Can you work these out from the model? Positions are in its coordinate system, mm. A direction names the side the tool comes from. Give positions to 0.01 mm unless a question says otherwise; leave off trailing zeros. Loops run counter-clockwise (first coordinate to the right, second up) from the corner with the lowest first, then second, coordinate; pieces in that order, holes last. Notation, with made-up numbers: (-22, 1.5) -> (-10, 1.5) arc R20 cw to (-10, 7.5) -> close; hole circle Ø10 at (45.5, 72.5). An arc over 180 degrees is marked (long way). Use CSV: the item, a comma, the result in double quotes.
from build123d import *

# Parameters (mm, degrees)
F3_DEPTH  = 6.501
F5_DEPTH  = 50
F8_W      = 9.4140861183
F8_H      = 9.8263791297
F9_DEPTH  = 25
F12_W     = 14.8912463337
F12_H     = 11.3480030559
F13_DEPTH = 25


with BuildPart() as f1:
    # F0 (on Front) → F1 (revolve)
    with BuildSketch(Plane.XZ):
        Polygon((-12, 5), (-22.5, 5), (-22.5, 5.6), (-23, 5.6), (-24.5, 5), (-24.5, 2.5), (-10, 2.5), (-8, 4.5), (-1, 4.5), (0, 5.5), (0, 6.5), (-10.5, 6.5), align=None)
    revolve(axis=Axis((-0.2357512317, 0, 0), (1, 0, 0)))

    # F2 (on Front) → F3 (cut, through all)
    with BuildSketch(Plane.XZ):
        with BuildLine():
            Line((0, 2.4), (-3.6575932294, 1.75))
            ThreePointArc((-3.6575932294, 1.75), (-7.7, 0), (-3.6575932294, -1.75))
            Line((-3.6575932294, -1.75), (0, -2.4))
            Line((0, -2.4), (0, 2.4))
        make_face()
    extrude(amount=-F3_DEPTH, mode=Mode.SUBTRACT)

    # F4 (on Top) → F5 (cut, symmetric)
    with BuildSketch(Plane.XY):
        with BuildLine():
            Line((-15.5885848908, 1.2395342523), (-24.5, 2.4))
            Line((-24.5, 2.4), (-24.5, -2.4))
            Line((-24.5, -2.4), (-15.5885848908, -1.2395342523))
            ThreePointArc((-15.5885848908, -1.2395342523), (-14.5, 0), (-15.5885848908, 1.2395342523))
        make_face()
    extrude(amount=F5_DEPTH, both=True, mode=Mode.SUBTRACT)

    # F8 (on 3pt) → F9 (cut)
    with BuildSketch(Plane(origin=(-0.2560212454, -0.0401067578, -5.558750384), x_dir=(0.9989411003, -0.0003319376, -0.046006173), z_dir=(0.0460073704, 0.0072072396, 0.9989151003))):
        with Locations((-24.0980023518, 1.025695703)):
            Rectangle(F8_W, F8_H)
    extrude(amount=-F9_DEPTH, mode=Mode.SUBTRACT)

    # F12 (on 3pt) → F13 (cut)
    with BuildSketch(Plane(origin=(-0.2560212454, -0.0401067578, 5.558750384), x_dir=(0.9989411003, -0.0003319376, 0.046006173), z_dir=(0.0460073704, 0.0072072396, -0.9989151003))):
        with Locations((-25.9663937613, -0.8096385282)):
            Rectangle(F12_W, F12_H)
    extrude(amount=-F13_DEPTH, mode=Mode.SUBTRACT)


solid = f1.part
(1) Which directions (+Z, -Z, +X, -X, +Y, -Y) give clear straight access to the entire face, cutting with the end or side of a thin tool? Please do faces 5 (the face through (-4.45, -4.46, -0.59)), 6 (the face through (-20.11, -1.83, 3.26)), 7 (the face through (-22.8, 5.6, -0.1)), 8 (the face through (-1.85, 5.07, -2.07)), 9 (the face through (-5.323, -6.445, -0.846)).
Answer sheet:
face 5,"+X"
face 6,"+Z, -Z, -X"
face 7,"-X, +Y"
face 8,"+X, +Y"
face 9,"+X, -X"
(2) If I drill on L1, parallel to Y at x = -21, z = 0; L2, parallel to Z at x = -2.5, y = 0; L3, parallel to Z at x = -4.75, y = 5.25, over which ranges is the centre line in solid material (lowest first)? Write a range as from..to.
Answer sheet:
L1,"y = -5..-2.5, 2.5..5"
L2,"z = -6.5..-4.5, 4.5..6.5"
L3,"z = -3.83..-2.34, 2.34..3.83"
(3) If we section it at D-D, the plane x = -13.5: Write out the boundary of the cut face in (y, z), then the cut area to 3 significant figures.
Answer sheet:
outline,"circle Ø10 at (0, 0); hole circle Ø5 at (0, 0)"
area,"58.9 mm2"
(4) If we section it at A-A, the plane y = 0: Write out the boundary of the cut face in (x, z), then the cut area to 4 significant figures.
Answer sheet:
outline,"(-14.5, -5) -> (-12, -5) -> (-10.5, -6.5) -> (0, -6.5) -> (0, -5.5) -> (-1, -4.5) -> (-8, -4.5) -> (-10, -2.5) -> (-14.5, -2.5) -> close; (-14.5, 2.5) -> (-10, 2.5) -> (-8, 4.5) -> (-1, 4.5) -> (0, 5.5) -> (0, 6.5) -> (-10.5, 6.5) -> (-12, 5) -> (-14.5, 5) -> close"
area,"69.25 mm2"
(5) If we section it at C-C, the plane x = -21: Write out the boundary of the cut face in (y, z).
Answer sheet:
outline,"(-1.98, -4.59) -> (-1.94, -4.59) -> (-1.94, -1.57) arc R2.5 cw to (-1.94, 1.57) -> (-1.94, 4.59) -> (-1.98, 4.59) arc R5 ccw to start; (1.94, -4.61) arc R5 ccw to (1.94, 4.61) -> (1.94, 1.57) arc R2.5 cw to (1.94, -1.57) -> close"
(6) Will these pins go through, and if not, where does the flat tip stop? pin 1 Ø6 at (x, y) = (-5, -5) entering from -Z; pin 2 Ø2 at (x, z) = (-14.5, -4) entering from -Y; pin 3 Ø5 at (y, z) = (1, 2) entering from +X; pin 4 Ø2 at (y, z) = (4, 3) entering from +X.
Answer sheet:
pin 1,"stops at z = -6.18"
pin 2,"stops at y = -4"
pin 3,"stops at x = -0.76"
pin 4,"stops at x = 0"
(7) We'd pull the mould along X, two halves only. Please class faces 1 (the face through (-22.5, -5.2, -0.3)), 2 (the face through (-0.826, -4.67, 0.176)), 3 (the face through (-17.324, 1.915, 4.619)), 4 (the face through (-24.094, 5.162, -0.078)): released by +X, released by -X, zero draft, split by the parting line, or undercut.
Answer sheet:
face 1,"undercut"
face 2,"released by +X"
face 3,"undercut"
face 4,"released by -X"
(8) If we section it at B-B, the plane z = 0: Write out the boundary of the cut face in (x, y).
Answer sheet:
outline,"(-24.5, -5) -> (-23, -5.6) -> (-22.5, -5.6) -> (-22.5, -5) -> (-12, -5) -> (-10.5, -6.5) -> (0, -6.5) -> (0, -5.5) -> (-1, -4.5) -> (-8, -4.5) -> (-10, -2.5) -> (-24.5, -2.5) -> close; (-24.5, 2.5) -> (-10, 2.5) -> (-8, 4.5) -> (-7.7, 4.5) -> (-7.7, 6.5) -> (-10.5, 6.5) -> (-12, 5) -> (-22.5, 5) -> (-22.5, 5.6) -> (-23, 5.6) -> (-24.5, 5) -> close"
